from build123d import *

# Parameters (mm, degrees)
F0_W      = 80
F0_H      = 19.25
F0_W_2    = 74.05
F0_H_2    = 11.1
F1_DEPTH  = 45
F0_W_3    = 9.63
F0_H_3    = 6
F2_DEPTH  = 14
F0_R      = 2.745
F3_DEPTH  = 8
F5_W      = 4
F5_H      = 29.0582341515
F6_DEPTH  = 3.07077
F5_H_2    = 15.9417658485
F7_DEPTH  = 8.2825263962
F11_R     = 3.5
F11_R_2   = 1.85
F12_DEPTH = 2
F13_DEPTH = 25


with BuildPart() as f1:
    # F0 (on Front) → F1 (new body)
    with BuildSketch(Plane.XZ):
        with Locations((-22.1932545304, 37.9297346771)):
            Rectangle(F0_W, F0_H)
        with Locations((-21.8290186286, 37.9297346771)):
            Rectangle(F0_W_2, F0_H_2, mode=Mode.SUBTRACT)
    extrude(amount=F1_DEPTH)

    # F0 (on Front) → F2 (join)
    with BuildSketch(Plane.XZ):
        with Locations((-21.8290186286, 37.9297346771)):
            Rectangle(F0_W_2, F0_H_2)
        with Locations((-21.8290186286, 37.9297346771)):
            Rectangle(F0_W_3, F0_H_3, mode=Mode.SUBTRACT)
    extrude(amount=F2_DEPTH)

    # F0 (on Front) → F3 (join)
    with BuildSketch(Plane.XZ):
        with Locations((-21.8290186286, 37.9297346771)):
            Rectangle(F0_W_3, F0_H_3)
        with Locations((-21.8290186286, 37.9297346771)):
            Circle(F0_R, mode=Mode.SUBTRACT)
    extrude(amount=F3_DEPTH)

    # F5 (on offset) → F6 (cut)
    with BuildSketch(Plane(origin=(0, 0, 28.3047346771), x_dir=(1, 0, 0), z_dir=(0, 0, -1))):
        with Locations((-22.1932545304, 30.4708829243)):
            Rectangle(F5_W, F5_H)
    extrude(amount=-F6_DEPTH, mode=Mode.SUBTRACT)

    # F5 (on offset) → F7 (cut)
    with BuildSketch(Plane(origin=(0, 0, 28.3047346771), x_dir=(1, 0, 0), z_dir=(0, 0, -1))):
        with Locations((-22.1932545304, 30.4708829243)):
            Rectangle(F5_W, F5_H)
        with Locations((-22.1932545304, 7.9708829243)):
            Rectangle(F5_W, F5_H_2)
    extrude(amount=-F7_DEPTH, mode=Mode.SUBTRACT)

    # F11 (on offset) → F12 (cut)
    with BuildSketch(Plane.XZ.offset(14)):
        with Locations((-50.5927884306, 38.0425482406)):
            Circle(F11_R)
        with Locations((-50.5927884306, 38.0425482406)):
            Circle(F11_R_2, mode=Mode.SUBTRACT)
        with Locations((0, 38.4429908707)):
            Circle(F11_R)
        with Locations((0, 38.4429908707)):
            Circle(F11_R_2, mode=Mode.SUBTRACT)
    extrude(amount=-F12_DEPTH, mode=Mode.SUBTRACT)

    # F13 (cut): faces of the model
    f13_faces = [f1.faces().sort_by_distance(p)[0] for p in [
        (0, -14, 38.4429908707),
        (-50.5927884306, -14, 38.0425482406),
    ]]
    extrude(f13_faces, amount=-F13_DEPTH, mode=Mode.SUBTRACT)


solid = f1.part
Design review of the part built by this model. Coordinates are the model's own, in mm. A direction names the side the tool comes from. Round coordinates to 2 decimals unless told otherwise and drop trailing zeros. Loops run counter-clockwise (first coordinate to the right, second up) from the corner with the lowest first, then second, coordinate; pieces in that order, holes last. Notation, with made-up numbers: (-25, -14.75) - (27, -14.75) arc R19 ccw to (27, -5.75) - close; hole circle Ø10 at (-5.75, 89.25). An arc over 180 degrees is marked (long way). One line per item, written item: value. Start each with the question number.
1) Consider section D-D on y = -11. Give the boundary of the cut face in (x, z).
2) Insertion check: pin 1 Ø7.5 at (x, z) = (-49.5, 37.5) entering from -Y; pin 2 Ø6.5 at (x, z) = (0, 38.44) entering from -Y. Each pin has a flat end and moves straight along its axis. Give the tip position at first contact, or say it passes through.
3) Consider section A-A on x = 0. Give the boundary of the cut face in (y, z), then the cut area to 3 significant figures.
4) To check wall thickness, follow L1, parallel to X at y = -36, z = 37.5; L2, parallel to X at y = -21.5, z = 29; L3, parallel to Z at x = -48.5, y = -37. State the ranges of each line that lie inside material, in increasing order. Write a range as from..to.
5) Consider section B-B on y = -41. Give the boundary of the cut face in (x, z), then the cut area to 3 significant figures.
6) For faces 1 (the flat face through (-58.854, -29, 38)), 2 (the cylindrical face through (-21.2, -3.9, 40.6)), list the 3-axis set-ups (+Z, -Z, +X, -X, +Y, -Y) from which the entire face can be reached by the end or side of a thin tool; tool diameter is ignored.
7) Consider section C-C on x = -43. Give the boundary of the cut face in (y, z).
8) Draft analysis for pull direction Z (two halves, no side actions). For faces 3 (the flat face through (-22, -14, 42)), 4 (the flat face through (-1, -22, 28.305)), 5 (the flat face through (17.807, -22, 38)), state which applies: +Z half, -Z half, draft (parallel to the pull), parting line (faces both ways), or undercut.
Reported:
1. outline: (-62.19, 28.3) - (-24.19, 28.3) - (-24.19, 34.93) - (-26.64, 34.93) - (-26.64, 40.93) - (-17.01, 40.93) - (-17.01, 34.93) - (-20.19, 34.93) - (-20.19, 28.3) - (17.81, 28.3) - (17.81, 47.55) - (-62.19, 47.55) - close; hole circle Ø3.7 at (-50.59, 38.04); hole circle Ø3.7 at (0, 38.44)
2. pin 1: stops at y = -14
2. pin 2: stops at y = -12
3. outline: (-45, 28.3) - (0, 28.3) - (0, 36.59) - (-12, 36.59) - (-12, 34.94) - (-14, 34.94) - (-14, 32.38) - (-45, 32.38) - close; (-45, 43.48) - (-14, 43.48) - (-14, 41.94) - (-12, 41.94) - (-12, 40.29) - (0, 40.29) - (0, 47.55) - (-45, 47.55) - close
3. area: 464 mm^2
4. L1: x = -62.19..-58.85, 15.2..17.81
4. L2: x = -62.19..-24.19, -20.19..17.81
4. L3: z = 28.3..32.38, 43.48..47.55
5. outline: (-62.19, 28.3) - (-24.19, 28.3) - (-24.19, 32.38) - (-58.85, 32.38) - (-58.85, 43.48) - (15.2, 43.48) - (15.2, 32.38) - (-20.19, 32.38) - (-20.19, 28.3) - (17.81, 28.3) - (17.81, 47.55) - (-62.19, 47.55) - close
5. area: 702 mm^2
6. face 1: -Y
6. face 2: +Y, -Y
7. outline: (-45, 28.3) - (0, 28.3) - (0, 47.55) - (-45, 47.55) - (-45, 43.48) - (-14, 43.48) - (-14, 32.38) - (-45, 32.38) - close
8. face 3: undercut
8. face 4: -Z half
8. face 5: draft
